Geometry: final body of the model. Coordinates: model frame, mm. Round coordinates to 2 decimals unless told otherwise and drop trailing zeros. Loops run counter-clockwise (first coordinate to the right, second up) from the corner with the lowest first, then second, coordinate; pieces in that order, holes last. Notation, with made-up numbers: M 9.25,82 L 65.25,82 A24 ccw 65.25,93 Z; hole C -31,-23.5 d3. An arc over 180 degrees is marked long. Answer as a JSON object with one key per item and string values.
from build123d import *

# Parameters (mm, degrees)
F0_R     = 11
F1_DEPTH = 3


with BuildPart() as f1:
    # F0 (on Front) → F1 (new body)
    with BuildSketch(Plane.XZ):
        with BuildLine():
            ThreePointArc((34.4457053252, 10.0615955075), (39.2169072518, 6.0040503586), (41, -2e-10))
            ThreePointArc((41, -2e-10), (39.218122302, -6.0021847046), (34.4497779591, -10.0597950337))
            add(Edge.make_bspline(
                [(34.4497779591, -10.0597950337), (33.5572864984, -14.2139641421), (32.0732731389, -17.7845741491), (30, -20)],
                knots=[0.5781750695, 0.5781750695, 0.5781750695, 0.5781750695, 0.6822186894, 0.6822186894, 0.6822186894, 0.6822186894], degree=3))
            ThreePointArc((30, -20), (50, 0), (30, 20))
            add(Edge.make_bspline(
                [(30, 20), (32.0727475467, 17.7685869814), (33.5539058525, 14.2021827738), (34.4457053252, 10.0615955075)],
                knots=[0.3177813106, 0.3177813106, 0.3177813106, 0.3177813106, 0.4213364669, 0.4213364669, 0.4213364669, 0.4213364669], degree=3))
        make_face()
        with BuildLine():
            ThreePointArc((34.4497779591, -10.0597950337), (19.0000002253, -0.0022264354), (34.4457053252, 10.0615955075))
            add(Edge.make_bspline(
                [(30, 20), (32.0727475467, 17.7685869814), (33.5539058525, 14.2021827738), (34.4457053252, 10.0615955075)],
                knots=[0.3177813106, 0.3177813106, 0.3177813106, 0.3177813106, 0.4213364669, 0.4213364669, 0.4213364669, 0.4213364669], degree=3))
            add(Edge.make_bspline(
                [(0, 15), (11.7076504976, 21.1235117167), (23.6393275279, 26.8475716609), (30, 20)],
                knots=[0, 0, 0, 0, 0.3177813106, 0.3177813106, 0.3177813106, 0.3177813106], degree=3))
            ThreePointArc((0, 15), (-6.7706330465, 13.3850113242), (-12.0833333333, 8.8878037532))
            ThreePointArc((-12.0833333333, 8.8878037532), (-19.4585597536, 16.9964124901), (-30, 20))
            add(Edge.make_bspline(
                [(-30, 20), (-32.0727475467, 17.7685869814), (-33.5539058525, 14.2021827738), (-34.4457053252, 10.0615955075)],
                knots=[0.3177813106, 0.3177813106, 0.3177813106, 0.3177813106, 0.4213364669, 0.4213364669, 0.4213364669, 0.4213364669], degree=3))
            ThreePointArc((-34.4457053252, 10.0615955075), (-23.9959496412, 9.2169072516), (-19, -2e-10))
            ThreePointArc((-19, -2e-10), (-23.9978152957, -9.2181223023), (-34.4497779591, -10.0597950337))
            add(Edge.make_bspline(
                [(-34.4497779591, -10.0597950337), (-33.5572864984, -14.2139641421), (-32.0732731389, -17.7845741491), (-30, -20)],
                knots=[0.5781750695, 0.5781750695, 0.5781750695, 0.5781750695, 0.6822186894, 0.6822186894, 0.6822186894, 0.6822186894], degree=3))
            add(Edge.make_bspline(
                [(-30, -20), (-23.6675842682, -26.7665939655), (-11.8380817304, -20.8909455716), (0, -15)],
                knots=[0.6822186894, 0.6822186894, 0.6822186894, 0.6822186894, 1, 1, 1, 1], degree=3))
            ThreePointArc((0, -15), (6.7706330465, -13.3850113242), (12.0833333333, -8.8878037532))
            ThreePointArc((12.0833333333, -8.8878037532), (19.4585597536, -16.9964124901), (30, -20))
            add(Edge.make_bspline(
                [(34.4497779591, -10.0597950337), (33.5572864984, -14.2139641421), (32.0732731389, -17.7845741491), (30, -20)],
                knots=[0.5781750695, 0.5781750695, 0.5781750695, 0.5781750695, 0.6822186894, 0.6822186894, 0.6822186894, 0.6822186894], degree=3))
        make_face()
        Circle(F0_R, mode=Mode.SUBTRACT)
        with BuildLine():
            add(Edge.make_bspline(
                [(-30, 20), (-32.0727475467, 17.7685869814), (-33.5539058525, 14.2021827738), (-34.4457053252, 10.0615955075)],
                knots=[0.3177813106, 0.3177813106, 0.3177813106, 0.3177813106, 0.4213364669, 0.4213364669, 0.4213364669, 0.4213364669], degree=3))
            ThreePointArc((-30, 20), (-50, 0), (-30, -20))
            add(Edge.make_bspline(
                [(-34.4497779591, -10.0597950337), (-33.5572864984, -14.2139641421), (-32.0732731389, -17.7845741491), (-30, -20)],
                knots=[0.5781750695, 0.5781750695, 0.5781750695, 0.5781750695, 0.6822186894, 0.6822186894, 0.6822186894, 0.6822186894], degree=3))
            ThreePointArc((-34.4497779591, -10.0597950337), (-40.9999997747, 0.0022264349), (-34.4457053252, 10.0615955075))
        make_face()
    extrude(amount=F1_DEPTH)


solid = f1.part
1) Pin query (flat end, axial travel): P1, Ø1.5, axis at y = -2.5, z = 2.5, coming from the -X side; P2, Ø17.5, axis at x = -30, z = 0, coming from the -Y side; P3, Ø1, axis at x = -18.5, y = -2.5, coming from the +Z side. Return the tip coordinate at first contact, or that it passes through.
Results:
{"P1": "x = -49.92", "P2": "through", "P3": "z = 16.7"}
2) Section query A-A (x = 39.5). Return the cut outline in (y, z).
Results:
{"outline": "M -3,-17.6 L 0,-17.6 L 0,-5.55 L -3,-5.55 Z; M -3,5.55 L 0,5.55 L 0,17.6 L -3,17.6 Z"}
3) Pull-direction query (Z, two-part tool) for faces 1 (the cylindrical face through (-2.38, -1.48, -10.74)), 2 (the flat face through (-12, -3, 0)); classes: +Z half, -Z half, draft (parallel to the pull), parting line (faces both ways), or undercut.
Results:
{"face 1": "undercut", "face 2": "draft"}
4) Section query C-C (y = -1.4). Count the separate pieces of the cut face and the enclosed holes in it, and give its area (3 significant figures).
Results:
{"separate pieces": "1", "enclosed holes": "3", "area": "2,270 mm2"}
5) Ray query, line 1 (Z direction, x = 30, y = -1.3); line 2 (Z direction, x = 0, y = -1.7); line 3 (X direction, y = -1.1, z = 1). Return the intervals inside material, ascending.
Results:
{"line 1": "-20 to -11, 11 to 20", "line 2": "-15 to -11, 11 to 15", "line 3": "-49.97 to -40.95, -19.05 to -10.95, 10.95 to 19.05, 40.95 to 49.97"}
6) Section query B-B (z = -5). Return the cut outline in (x, y).
Results:
{"outline": "M -49.36,-3 L -39.8,-3 L -39.8,0 L -49.36,0 Z; M -20.2,-3 L -9.8,-3 L -9.8,0 L -20.2,0 Z; M 9.8,-3 L 20.2,-3 L 20.2,0 L 9.8,0 Z; M 39.8,-3 L 49.36,-3 L 49.36,0 L 39.8,0 Z"}
